Build history of the part. All positions in model axes, mm. Face numbers are marked on the shaded views. Round coordinates to 2 decimals unless told otherwise and drop trailing zeros. Write each loop counter-clockwise with the first axis right and the second up, starting at its lowest first coordinate (ties: lowest second). Pieces come first, ordered by that corner, then holes.
1) Saw through at D-D (x = -13.5). Write the cut outline in (y, z).
2) Saw through at C-C (z = 17.5). Write the cut outline in (x, y), plus the area to 3 significant figures.
3) Saw through at A-A (x = 17). Write the cut outline in (y, z).
4) Wall check: probe 1 along Z at (x, y) = (10, 1.1); probe 2 along Z at (x, y) = (18.5, 1.8); probe 3 along X at (y, z) = (1.2, 6.5). Give the ranges that are in metal, low to high.
5) Flat gauge pins, fed straight in: pin 1 (3 mm diameter, centred on x = 15, z = 14, fed in from -Y); pin 2 (0.9 mm diameter, centred on x = 5.5, y = 1, fed in from -Z); pin 3 (0.9 mm diameter, centred on x = 7.5, y = 2, fed in from +Z); pin 4 (1 mm diameter, centred on x = 17, y = 0.5, fed in from -Z). Where does each tip first touch, or does it go through?
6) Pull direction Z, two halves, no side cores. Call the marked faces 1, 2 and 3: +Z half, -Z half, draft (parallel to the pull), parting line (faces both ways), or undercut.
from build123d import *

# Parameters (mm, degrees)
BOSS_EXTRUDE1_DEPTH = 3


with BuildPart() as part:
    # Sketch1 → Boss-Extrude1 (new body)
    with BuildSketch(Plane(origin=(0, 0, 0), x_dir=(1, 0, 0), z_dir=(0, 1, 0))):
        with BuildLine():
            Line((21.125095664, -3.9), (0, -3.9))
            ThreePointArc((0, -3.9), (-3.9, 0), (0, 3.9))
            Line((0, 3.9), (21.125095664, 3.9))
            ThreePointArc((21.125095664, 3.9), (21.134212017, 3.899989345), (21.14332832, 3.899957381))
            ThreePointArc((21.14332832, 3.899957381), (-21.5, 0), (21.14332832, -3.899957381))
            ThreePointArc((21.14332832, -3.899957381), (21.134212017, -3.899989345), (21.125095664, -3.9))
        make_face()
    extrude(amount=BOSS_EXTRUDE1_DEPTH)


solid = part.part
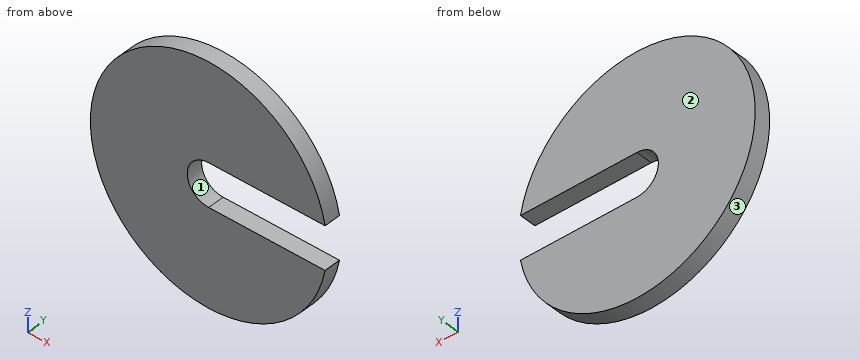
Evaluation:
1. outline: (0, -16.73) - (3, -16.73) - (3, 16.73) - (0, 16.73) - close
2. outline: (-12.49, 0) - (12.49, 0) - (12.49, 3) - (-12.49, 3) - close
2. area: 74.9 mm2
3. outline: (0, -13.16) - (3, -13.16) - (3, -3.9) - (0, -3.9) - close; (0, 3.9) - (3, 3.9) - (3, 13.16) - (0, 13.16) - close
4. probe 1: z = -19.03 to -3.9, 3.9 to 19.03
4. probe 2: z = -10.95 to -3.9, 3.9 to 10.95
4. probe 3: x = -20.49 to 20.49
5. pin 1: stops at y = 0
5. pin 2: stops at z = -20.9
5. pin 3: stops at z = 20.31
5. pin 4: stops at z = -13.78
6. face 1: undercut
6. face 2: draft
6. face 3: parting line
